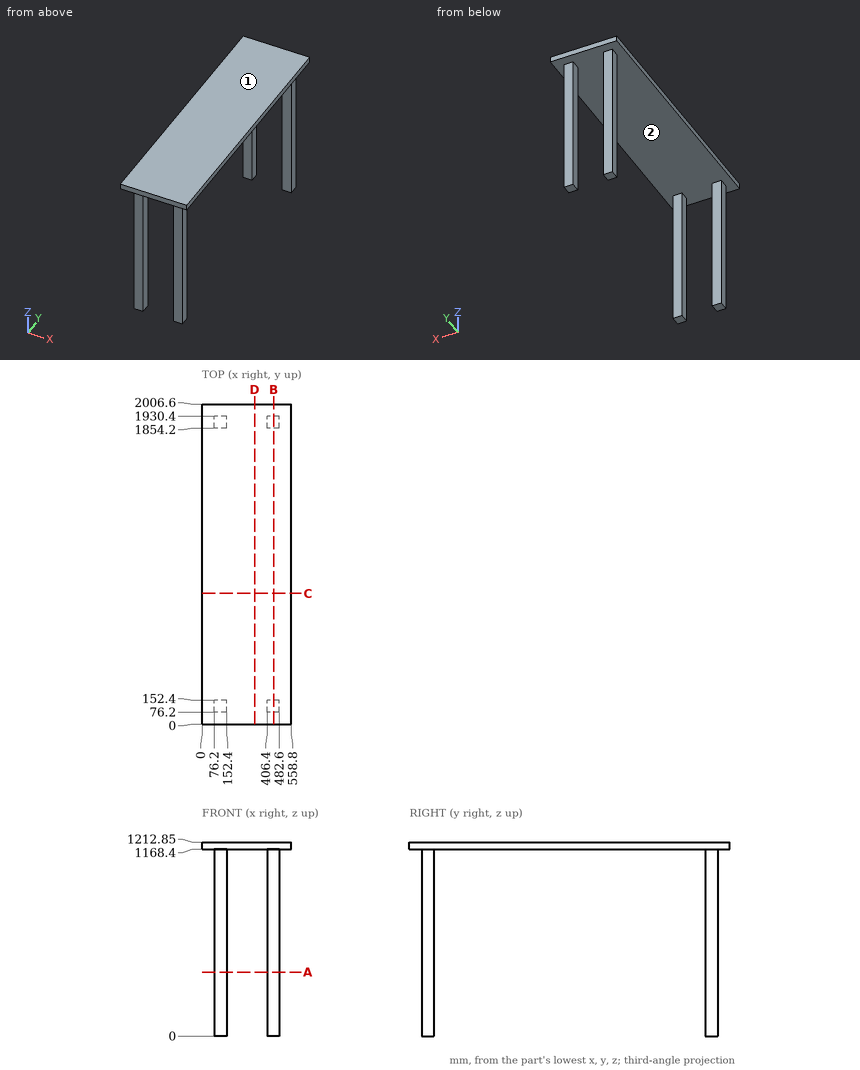
Input: dimensioned drawing with shaded views. Units: mm. Origin: part minimum x, y, z. Coordinates: 2 decimals unless noted, no trailing zeros. Order: outer loops, then holes, each group sorted by start corner. A loop starts at its lowest first (then second) coordinate and runs counter-clockwise, first axis right, second up.
1. Cut plane A-A, the plane z = 400. Return loops of the section in (x, y).
Checked values:
outline: (76.2, 76.2) - (152.4, 76.2) - (152.4, 152.4) - (76.2, 152.4) - close; (76.2, 1854.2) - (152.4, 1854.2) - (152.4, 1930.4) - (76.2, 1930.4) - close; (406.4, 76.2) - (482.6, 76.2) - (482.6, 152.4) - (406.4, 152.4) - close; (406.4, 1854.2) - (482.6, 1854.2) - (482.6, 1930.4) - (406.4, 1930.4) - close
2. Cut plane B-B, the plane x = 447. Return loops of the section in (y, z).
Checked values:
outline: (0, 1168.4) - (76.2, 1168.4) - (76.2, 0) - (152.4, 0) - (152.4, 1168.4) - (1854.2, 1168.4) - (1854.2, 0) - (1930.4, 0) - (1930.4, 1168.4) - (2006.6, 1168.4) - (2006.6, 1212.85) - (0, 1212.85) - close
3. Contact query for flat-ended pins moving along their axis: P1, Ø4, axis at x = 97, z = 986, coming from the -Y side; P2, Ø3, axis at x = 468.5, z = 251.5, coming from the +Y side; P3, Ø23, axis at y = 131.5, z = 431.5, coming from the -X side. Output: stop coordinate, or through.
Checked values:
P1: stops at y = 76.2
P2: stops at y = 1930.4
P3: stops at x = 76.2
4. Ray query, line 1 along Y through (x, z) = (430.5, 94.5); line 2 along X through (y, z) = (1887.5, 237); line 3 along Z through (x, y) = (474, 987.5). Return the intervals inside material, ascending.
Checked values:
line 1: y = 76.2 to 152.4, 1854.2 to 1930.4
line 2: x = 76.2 to 152.4, 406.4 to 482.6
line 3: z = 1168.4 to 1212.85
5. Cut plane C-C, the plane y = 820.5. Return loops of the section in (x, z), plus the area to 3 significant figures.
Checked values:
outline: (0, 1168.4) - (558.8, 1168.4) - (558.8, 1212.85) - (0, 1212.85) - close
area: 24,800 mm2
6. Cut plane D-D, the plane x = 328. Return loops of the section in (y, z), plus the area to 3 significant figures.
Checked values:
outline: (0, 1168.4) - (2006.6, 1168.4) - (2006.6, 1212.85) - (0, 1212.85) - close
area: 89,200 mm2
7. Draft query along Y for the marked faces 1 and 2. Return one class per face: +Y half, -Y half, draft (parallel to the pull), parting line (faces both ways), or undercut.
Checked values:
face 1: draft
face 2: undercut
